Read the model definition and answer for the solid it produces. Units are mm, in the model's axes. Face numbers are marked on the shaded views. A direction names the side the tool comes from. Round coordinates to 2 decimals unless told otherwise and drop trailing zeros. Order: outer loops, then holes, each group sorted by start corner. A loop starts at its lowest first (then second) coordinate and runs counter-clockwise, first axis right, second up. Notation, with made-up numbers: (29.5, 45) -> (35.5, 45) arc R24 cw to (35.5, 67) -> close; hole circle Ø11 at (16, 65.25). An arc over 180 degrees is marked (long way). Use a Markdown table: item, result. Add a question column.
1. Section A-A, the plane x = -1 is taken. Give the vertices of the cut face in (y, z), then the cut area to 3 significant figures.
2. The mould has two halves that part along Y. Classify the marked faces 5, 6 and 7: +Y half, -Y half, draft (parallel to the pull), parting line (faces both ways), or undercut.
3. For the marked faces 1, 2, 3 and 4, determine the directions among +Z, -Z, +X, -X, +Y, -Y from which every point of the face is accessible in a straight line to the end or side of a thin tool.
4. Section C-C, the plane z = 6 is taken. Give the number of separate pieces and of enclosed holes in the cut face, then the cut area to 3 significant figures.
5. Section D-D, the plane y = -12.5 is taken. Give the vertices of the cut face in (x, z), then the cut area to 3 significant figures.
6. Consider L1, parallel to Y at x = -8, z = 3.5; L2, parallel to Y at x = 0, z = 16.15; L3, parallel to Z at x = 0, y = 1. Determine where each line is inside the solid, lowest interval first. Write a range as [from, to].
7. Given pin 1 (4 mm diameter, centred on x = 5.5, z = 3.5, fed in from +Y); pin 2 (9 mm diameter, centred on x = 6, z = 4.5, fed in from +Y); pin 3 (9 mm diameter, centred on x = 4, z = 5, fed in from +Y), each flat-ended and moving along its own axis, determine where each tip first touches the part or whether it passes through.
8. Section B-B, the plane y = -3 is taken. Give the vertices of the cut face in (x, z), then the cut area to 3 significant figures.
```python
from build123d import *

# Parameters (mm, degrees)
F0_R          = 16
F1_DEPTH      = 20
F3_DEPTH      = 25
F5_DEPTH      = 16.001
F5_DEPTH_BACK = 16.001
F6_R          = 14.05
F7_DEPTH      = 5
F8_W          = 10.4940169359
F8_H          = 10.4940169359
F9_DEPTH      = 10.92124


with BuildPart() as f1:
    # F0 (on Top) → F1 (new body)
    with BuildSketch(Plane.XY):
        Circle(F0_R)
    extrude(amount=F1_DEPTH)

    # F2 (on Front) → F3 (cut, symmetric)
    with BuildSketch(Plane.XZ):
        Polygon((16, 8.237604307), (10.6666666667, -1), (21.3333333333, -1), align=None)
        Polygon((5.3333333333, 8.237604307), (0, -1), (10.6666666667, -1), align=None)
        Polygon((-5.3333333333, 8.237604307), (-10.6666666667, -1), (0, -1), align=None)
        Polygon((-16, 8.237604307), (-21.3333333333, -1), (-10.6666666667, -1), align=None)
    extrude(amount=F3_DEPTH, both=True, mode=Mode.SUBTRACT)

    # F4 (on Right) → F5 (cut, two sides)
    with BuildSketch(Plane.YZ) as f5_sk:
        Polygon((16, 8.237604307), (10.6666666667, -1), (21.3333333333, -1), align=None)
        Polygon((5.3333333333, 8.237604307), (0, -1), (10.6666666667, -1), align=None)
        Polygon((-5.3333333333, 8.237604307), (-10.6666666667, -1), (0, -1), align=None)
        Polygon((-16, 8.237604307), (-21.3333333333, -1), (-10.6666666667, -1), align=None)
    extrude(amount=-F5_DEPTH, mode=Mode.SUBTRACT)
    extrude(f5_sk.sketch, amount=F5_DEPTH_BACK, mode=Mode.SUBTRACT)

    # F6 (on face) → F7 (cut)
    with BuildSketch(Plane.XY.offset(20)):
        Circle(F6_R)
    extrude(amount=-F7_DEPTH, mode=Mode.SUBTRACT)

    # F8 (on Top) → F9 (join)
    with BuildSketch(Plane.XY):
        Polygon((-11.2440169359, -11.2440169359), (11.2440169359, -11.2440169359), (11.2440169359, -10.7440169359), (11.2440169359, -0.25), (11.2440169359, 0.25), (11.2440169359, 10.7440169359), (11.2440169359, 11.2440169359), (-11.2440169359, 11.2440169359), (-11.2440169359, 10.7440169359), (-11.2440169359, 0.25), (-11.2440169359, -0.25), (-11.2440169359, -10.7440169359), align=None)
        with Locations((-5.4970084679, -5.4970084679)):
            Rectangle(F8_W, F8_H, mode=Mode.SUBTRACT)
        with Locations((5.4970084679, -5.4970084679)):
            Rectangle(F8_W, F8_H, mode=Mode.SUBTRACT)
        with Locations((-5.4970084679, 5.4970084679)):
            Rectangle(F8_W, F8_H, mode=Mode.SUBTRACT)
        with Locations((5.4970084679, 5.4970084679)):
            Rectangle(F8_W, F8_H, mode=Mode.SUBTRACT)
    extrude(amount=F9_DEPTH)


solid = f1.part
```
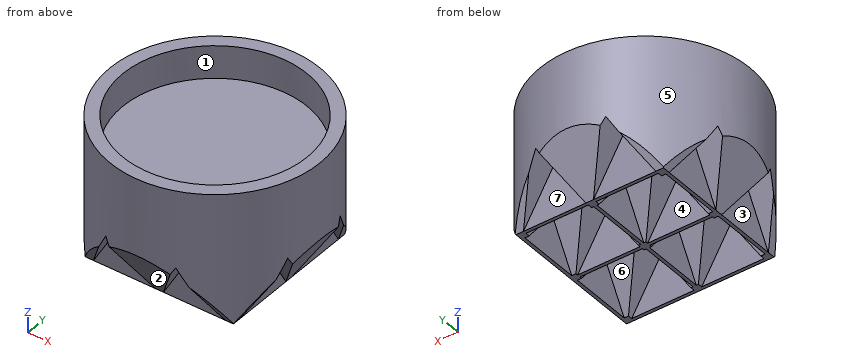
Verdict:
| question | item | result |
|---|---|---|
| 1 | outline | (-15.97, 8.18) -> (-11.67, 0.73) -> (-11.24, 0.73) -> (-11.24, 0) -> (-10.74, 0) -> (-10.74, 0.73) -> (-9.67, 0.73) -> (-5.33, 8.24) -> (-1, 0.73) -> (-0.25, 0.73) -> (-0.25, 0) -> (0.25, 0) -> (0.25, 0.73) -> (1, 0.73) -> (5.33, 8.24) -> (9.67, 0.73) -> (10.74, 0.73) -> (10.74, 0) -> (11.24, 0) -> (11.24, 0.73) -> (11.67, 0.73) -> (15.97, 8.18) -> (15.97, 20) -> (14.01, 20) -> (14.01, 15) -> (-14.01, 15) -> (-14.01, 20) -> (-15.97, 20) -> close |
| 1 | area | 379 mm2 |
| 2 | face 5 | parting line |
| 2 | face 6 | undercut |
| 2 | face 7 | +Y half |
| 3 | face 1 | +Z |
| 3 | face 2 | -Z, +X, -X, -Y |
| 3 | face 3 | -Z, -X |
| 3 | face 4 | -Z |
| 4 | separate pieces | 1 |
| 4 | enclosed holes | 4 |
| 4 | area | 499 mm2 |
| 5 | outline | (-9.99, 2.18) -> (-8.83, 2.18) -> (-5.33, 8.24) -> (-1.83, 2.18) -> (1.83, 2.18) -> (5.33, 8.24) -> (8.83, 2.18) -> (9.99, 2.18) -> (9.99, 20) -> (6.42, 20) -> (6.42, 15) -> (-6.42, 15) -> (-6.42, 20) -> (-9.99, 20) -> close |
| 5 | area | 249 mm2 |
| 6 | L1 | y = [-11.24, -10.74], [-0.25, 0.25], [10.74, 11.24] |
| 6 | L2 | y = [-16, -14.05], [14.05, 16] |
| 6 | L3 | z = [0, 15] |
| 7 | pin 1 | stops at y = 11.24 |
| 7 | pin 2 | stops at y = 15.73 |
| 7 | pin 3 | stops at y = 15.98 |
| 8 | outline | (-15.72, 7.75) -> (-13.67, 4.2) -> (-11.24, 4.2) -> (-11.24, 0) -> (-10.74, 0) -> (-10.74, 4.2) -> (-7.67, 4.2) -> (-5.33, 8.24) -> (-3, 4.2) -> (-0.25, 4.2) -> (-0.25, 0) -> (0.25, 0) -> (0.25, 4.2) -> (3, 4.2) -> (5.33, 8.24) -> (7.67, 4.2) -> (10.74, 4.2) -> (10.74, 0) -> (11.24, 0) -> (11.24, 4.2) -> (13.67, 4.2) -> (15.72, 7.75) -> (15.72, 20) -> (13.73, 20) -> (13.73, 15) -> (-13.73, 15) -> (-13.73, 20) -> (-15.72, 20) -> close |
| 8 | area | 340 mm2 |
